```python
from build123d import *

# Parameters (mm, degrees)
CUT_EXTRUDE1_START = 38.35654
CUT_EXTRUDE1_DEPTH = 2.02616
SKETCH4_R          = 1.833087105
CUT_EXTRUDE2_DEPTH = 1.02616
CUT_EXTRUDE2_DRAFT = -45


with BuildPart() as part:
    # Sketch2 → Revolve1 (revolve)
    with BuildSketch(Plane(origin=(0, 0, 0), x_dir=(0, 0, -1), z_dir=(1, 0, 0))):
        with BuildLine():
            Line((-39.3827, 1.5875), (-39.3827, 2.2225))
            ThreePointArc((-39.3827, 2.2225), (-38.467752118, 3.57733025), (-37.180157143, 4.5847))
            Line((-37.180157143, 4.5847), (-36.8173, 4.5847))
            Line((-36.8173, 4.5847), (-36.8173, 2.413))
            Line((-36.8173, 2.413), (38.7873875, 2.413))
            Line((38.7873875, 2.413), (39.3827, 1.8176875))
            Line((39.3827, 1.8176875), (39.3827, 0))
            Line((39.3827, 0), (-37.439996448, 0))
            Line((-37.439996448, 0), (-38.35654, 1.5875))
            Line((-38.35654, 1.5875), (-39.3827, 1.5875))
        make_face()
    revolve(axis=Axis((0, 0, 39.3827), (0, 0, -1)))

    # Sketch3 → Cut-Extrude1 (cut, through all)
    with BuildSketch(Plane.XY.offset(CUT_EXTRUDE1_START)):
        Polygon((0, 1.833087105), (-1.5875, 0.916543552), (-1.5875, -0.916543552), (0, -1.833087105), (1.5875, -0.916543552), (1.5875, 0.916543552), align=None)
    extrude(amount=CUT_EXTRUDE1_DEPTH, mode=Mode.SUBTRACT)


with BuildPart() as cut_extrude2_tool:
    # Sketch4 → Cut-Extrude2 (with draft: the straight prism first)
    with BuildSketch(Plane.XY.offset(39.3827)):
        Circle(SKETCH4_R)
    extrude(amount=-CUT_EXTRUDE2_DEPTH)
    # Cut-Extrude2: the draft: its side faces are tilted about the plane it starts from
    cut_extrude2_sides = [cut_extrude2_tool.faces().sort_by_distance(p)[0] for p in [
        (-1.833087105, 0, 38.86962),
    ]]
    draft(cut_extrude2_sides, Plane.XY.offset(39.3827), CUT_EXTRUDE2_DRAFT)


with BuildPart() as part_1:
    add(part.part)

    # Cut-Extrude2: cut by cut_extrude2_tool
    add(cut_extrude2_tool.part, mode=Mode.SUBTRACT)


solid = part_1.part
```
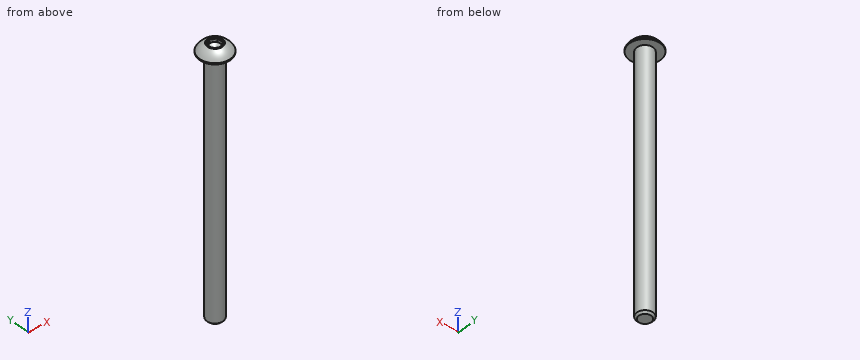
The model under review builds one solid part; all positions refer to its coordinate system, in mm. Coordinates: 2 decimals unless noted, no trailing zeros. Write each loop counter-clockwise with the first axis right and the second up, starting at its lowest first coordinate (ties: lowest second). Pieces come first, ordered by that corner, then holes. Notation, with made-up numbers: (36, 21) -> (57, 21) arc R20 cw to (57, 47) -> close; hole circle Ø7 at (-6, 50). An arc over 180 degrees is marked (long way). One line per item, written item: value. Start each with the question number.
Q1. Clearance check with flat-ended pins moving along their axes: P1, Ø1.5, axis at x = 1, z = -28.5, coming from the -Y side; P2, Ø1.1, axis at y = -0.5, z = 39, coming from the +X side; P3, Ø0.5, axis at y = 0.5, z = 39, coming from the -X side; P4, Ø0.6, axis at x = 1.5, y = -1, coming from the +Z side. State where each tip first meets the part, or that it passes through.
Q2. Add section B-B, the plane y = -3.25. Give the boundary of the cut face in (x, z), then the cut area to 3 significant figures.
Q3. Add section A-A, the plane z = 18.5. Give the boundary of the cut face in (x, y), then the cut area to 3 significant figures.
Q4. To check wall thickness, follow probe 1 along X at (y, z) = (-0.25, 35.5); probe 2 along X at (y, z) = (1.5, -5). State the ranges of each line that lie inside material, in increasing order.
Response:
1. P1: y = -2.4
1. P2: x = 3.57
1. P3: x = -3.21
1. P4: z = 39.38
2. outline: (-3.23, 36.82) -> (3.23, 36.82) -> (3.23, 37.18) arc R4.12 ccw to (-3.23, 37.18) -> close
2. area: 9.42 mm²
3. outline: circle Ø4.83 at (0, 0)
3. area: 18.3 mm²
4. probe 1: -2.4 to 2.4
4. probe 2: -1.89 to 1.89
